Part model, mm, in its own coordinate system. A direction names the side the tool comes from. Coordinates: 2 decimals unless noted, no trailing zeros. Loops run counter-clockwise (first coordinate to the right, second up) from the corner with the lowest first, then second, coordinate; pieces in that order, holes last. Notation, with made-up numbers: (-20.5, 28.25) - (5.5, 28.25) arc R18 ccw to (5.5, 53.25) - close; hole circle Ø3 at (72, 84). An arc over 180 degrees is marked (long way). Use a Markdown table: item, result. Add a question column.
1. Wall check: probe 1 along Y at (x, z) = (-36, 17); probe 2 along Y at (x, z) = (-6.5, 23); probe 3 along X at (y, z) = (6, 22.5). Give the ranges that are in metal, low to high. Write a range as [from, to].
2. Pull direction Y, two halves, no side cores. Call faces 1 (the flat face through (-16, -54.658, 12)), 2 (the flat face through (-65.155, 5, 12)), 3 (the flat face through (-16, 50, 10)): pulls with the +Y half, pulls with the -Y half, needs draft (parallel to the pull), parting line crosses it, or undercut.
3. Drop flat-ended pins along their axis: pin 1 (2.5 mm diameter, centred on x = 31.84, y = 58.34, fed in from +Z); pin 2 (1.6 mm diameter, centred on x = -62.16, y = 58.34, fed in from +Z); pin 3 (3 mm diameter, centred on x = -56, y = 49, fed in from +Z). Give the stop position or say it passes through.
4. Band-saw the part on C-C, the plane x = -6.5. Give the cut face in (y, z).
5. Band-saw the part on A-A, the plane x = 10.5. Give the cut face in (y, z), plus the area to 3 significant figures.
6. Band-saw the part on B-B, the plane y = 10. Give the cut face in (x, z), plus the area to 3 significant figures.
7. 3-axis set-ups, long thin cutter, end or side, ignore diameter. For faces 4 (the cylindrical face through (-57.153, 50.43, 3.549)), 5 (the flat face through (27, 50, 7)), 6 (the flat face through (-16, 40.342, 18)): which of +Z, -Z, +X, -X, +Y, -Y reach the whole face in a straight line?
8. Band-saw the part on D-D, the plane z = 3.5. Count the separate pieces of the cut face and the enclosed holes in it, plus the area to 3 significant figures.
from build123d import *

# Parameters (mm, degrees)
F0_W     = 100
F0_H     = 120
F0_R     = 10
F1_DEPTH = 25
F2_W     = 100
F2_H     = 20
F3_DEPTH = 15
F4_R     = 1
F4_R_2   = 5
F4_R_3   = 0.5
F5_DEPTH = 3
F6_R     = 2
F6_R_2   = 1
F7_DEPTH = 25


with BuildPart() as f1:
    # F0 (on Top) → F1 (new body)
    with BuildSketch(Plane.XY):
        with Locations((-15.155184, 5.342288)):
            Rectangle(F0_W, F0_H)
        with Locations((-15.155184, -34.657712)):
            Circle(F0_R, mode=Mode.SUBTRACT)
        with Locations((-15.155184, 5.342288)):
            Circle(F0_R, mode=Mode.SUBTRACT)
    extrude(amount=F1_DEPTH)

    # F2 (on face) → F3 (cut)
    with BuildSketch(Plane.XY.offset(25)):
        with Locations((-15.155184, 50.342288)):
            Rectangle(F2_W, F2_H)
    extrude(amount=-F3_DEPTH, mode=Mode.SUBTRACT)

    # F4 (on face) → F5 (cut)
    with BuildSketch(Plane.XY.offset(10)):
        with Locations((-62.155184, 58.342288)):
            Circle(F4_R)
        with Locations((-37.155184, 58.342288)):
            Circle(F4_R)
        with Locations((-55.155184, 50.342288)):
            Circle(F4_R_2)
        with Locations((-45.155184, 50.342288)):
            Circle(F4_R_3)
        with Locations((-35.155184, 30.333549)):
            Circle(F4_R_3)
        with Locations((-62.155184, 42.342288)):
            Circle(F4_R)
        with Locations((-37.155184, 42.342288)):
            Circle(F4_R)
        with Locations((31.844816, 58.342288)):
            Circle(F4_R)
        with Locations((6.844816, 58.342288)):
            Circle(F4_R)
        with Locations((24.844816, 50.342288)):
            Circle(F4_R_2)
        with Locations((31.844816, 42.342288)):
            Circle(F4_R)
        with Locations((6.844816, 42.342288)):
            Circle(F4_R)
        with Locations((14.844816, 50.342288)):
            Circle(F4_R_3)
        with Locations((4.844816, 30.333549)):
            Circle(F4_R_3)
    extrude(amount=-F5_DEPTH, mode=Mode.SUBTRACT)

    # F6 (on face) → F7 (cut)
    with BuildSketch(Plane.XY.offset(10)):
        with Locations((24.844816, 50.342288)):
            Circle(F6_R)
        with Locations((31.844816, 42.342288)):
            Circle(F6_R_2)
        with Locations((31.844816, 58.342288)):
            Circle(F6_R_2)
        with Locations((6.844816, 42.342288)):
            Circle(F6_R_2)
        with Locations((-37.155184, 42.342288)):
            Circle(F6_R_2)
        with Locations((-62.155184, 42.342288)):
            Circle(F6_R_2)
        with Locations((6.844816, 58.342288)):
            Circle(F6_R_2)
        with Locations((-37.155184, 58.342288)):
            Circle(F6_R_2)
        with Locations((-55.155184, 50.342288)):
            Circle(F6_R)
        with Locations((-62.155184, 58.342288)):
            Circle(F6_R_2)
    extrude(amount=-F7_DEPTH, mode=Mode.SUBTRACT)


solid = f1.part
Geometry check:
| question | item | result |
|---|---|---|
| 1 | probe 1 | y = [-54.66, 40.34], [60.34, 65.34] |
| 1 | probe 2 | y = [-54.66, -39.67], [-29.65, 0.33], [10.35, 40.34], [60.34, 65.34] |
| 1 | probe 3 | x = [-65.16, -25.13], [-5.18, 34.84] |
| 2 | face 1 | pulls with the -Y half |
| 2 | face 2 | needs draft |
| 2 | face 3 | undercut |
| 3 | pin 1 | stops at z = 10 |
| 3 | pin 2 | passes through |
| 3 | pin 3 | stops at z = 7 |
| 4 | outline | (-54.66, 0) - (-39.67, 0) - (-39.67, 25) - (-54.66, 25) - close; (-29.65, 0) - (0.33, 0) - (0.33, 25) - (-29.65, 25) - close; (10.35, 0) - (65.34, 0) - (65.34, 25) - (60.34, 25) - (60.34, 10) - (40.34, 10) - (40.34, 25) - (10.35, 25) - close |
| 5 | outline | (-54.66, 0) - (65.34, 0) - (65.34, 25) - (60.34, 25) - (60.34, 10) - (40.34, 10) - (40.34, 25) - (-54.66, 25) - close |
| 5 | area | 2,700 mm^2 |
| 6 | outline | (-65.16, 0) - (-24, 0) - (-24, 25) - (-65.16, 25) - close; (-6.31, 0) - (34.84, 0) - (34.84, 25) - (-6.31, 25) - close |
| 6 | area | 2,060 mm^2 |
| 7 | face 4 | +Z, -Z |
| 7 | face 5 | +Z |
| 7 | face 6 | +Z, +X, -X |
| 8 | separate pieces | 1 |
| 8 | enclosed holes | 12 |
| 8 | area | 11,300 mm^2 |
